For this review, take the finished solid that the model builds, in its own axes (mm). A direction names the side the tool comes from. Round coordinates to 2 decimals unless told otherwise and drop trailing zeros. Loops run counter-clockwise (first coordinate to the right, second up) from the corner with the lowest first, then second, coordinate; pieces in that order, holes last.
1. To check wall thickness, follow line 1 along Y through (x, z) = (-15.5, 0.2); line 2 along Y through (x, z) = (-35, 1.4); line 3 along X through (y, z) = (-39.5, 1.95). State the ranges of each line that lie inside material, in increasing order.
2. Clearance check with a flat-ended pin moving along its axis: pin 1 Ø1 at (x, z) = (34, 0.5) entering from +Y. State where the tip first meets the part, or that it passes through.
3. Tool access review of faces 1 (the flat face through (-69, 24.134, 2)), 2 (the cylindrical face through (-3.96, 39.67, 1.57)): name each direction out of +Z, -Z, +X, -X, +Y, -Y from which nothing blocks a thin tool from reaching the whole face with its end or side.
4. Consider section C-C on x = 26. State the section outline as (y, z) points (3 decimals), then the cut area to 3 significant figures.
5. Consider section D-D on y = 28. State the section outline as (x, z) points (3 decimals), then the cut area to 3 significant figures.
6. Draft analysis for pull direction Y (two halves, no side actions). For faces 3 (the cylindrical face through (49.284, -2.851, 1.565)), 4 (the flat face through (2, -1, 0)), 5 (the cylindrical face through (-53.986, 22.745, 1.565)), state which applies: released by +Y, released by -Y, zero draft, split by the parting line, or undercut.
7. Consider section B-B on z = 2.4. State how many separate pieces and enclosed holes the cut face has, then the cut area to 3 significant figures.
8. Consider section A-A on y = -7. State the section outline as (x, z) points (3 decimals).
from build123d import *

# Parameters (mm, degrees)
SKETCH1_R           = 64.5
SKETCH1_R_2         = 1.65
SKETCH1_R_3         = 13
SKETCH1_R_4         = 1.4
BOSS_EXTRUDE2_DEPTH = 3.175
CUT_EXTRUDE1_DEPTH  = 3.175


with BuildPart() as part:
    # Sketch1 → Boss-Extrude2 (new body)
    with BuildSketch(Plane(origin=(0, 0, 0), x_dir=(-1, 0, 0), z_dir=(0, 0, 1))):
        with Locations((15.168596538, 0.366425758)):
            Circle(SKETCH1_R)
        with Locations((15.168596538, -60.283574242)):
            Circle(SKETCH1_R_2, mode=Mode.SUBTRACT)
        with Locations((15.168596538, 61.016425758)):
            Circle(SKETCH1_R_2, mode=Mode.SUBTRACT)
        with Locations((26.018596538, -38.058574242)):
            Circle(SKETCH1_R_2, mode=Mode.SUBTRACT)
        with Locations((4.318596538, -38.058574242)):
            Circle(SKETCH1_R_2, mode=Mode.SUBTRACT)
        with Locations((26.018596538, 38.791425758)):
            Circle(SKETCH1_R_2, mode=Mode.SUBTRACT)
        with Locations((4.318596538, 38.791425758)):
            Circle(SKETCH1_R_2, mode=Mode.SUBTRACT)
        with Locations((15.168596538, 0.366425758)):
            Circle(SKETCH1_R_3, mode=Mode.SUBTRACT)
        with Locations((54.168596538, -24.133574242)):
            Circle(SKETCH1_R_4, mode=Mode.SUBTRACT)
        with Locations((54.168596538, 24.866425758)):
            Circle(SKETCH1_R_4, mode=Mode.SUBTRACT)
        with Locations((-3.831403462, -24.133574242)):
            Circle(SKETCH1_R_4, mode=Mode.SUBTRACT)
        with Locations((-3.831403462, 24.866425758)):
            Circle(SKETCH1_R_4, mode=Mode.SUBTRACT)
        with Locations((-5.831403462, 56.366425758)):
            Circle(SKETCH1_R_2, mode=Mode.SUBTRACT)
        with Locations((-22.394874657, 46.366425758)):
            Circle(SKETCH1_R_2, mode=Mode.SUBTRACT)
        with Locations((36.168596538, 56.366425758)):
            Circle(SKETCH1_R_2, mode=Mode.SUBTRACT)
        with Locations((52.732067734, 46.366425758)):
            Circle(SKETCH1_R_2, mode=Mode.SUBTRACT)
        with Locations((52.732067734, -45.633574242)):
            Circle(SKETCH1_R_2, mode=Mode.SUBTRACT)
        with Locations((36.168596538, -55.633574242)):
            Circle(SKETCH1_R_2, mode=Mode.SUBTRACT)
        with Locations((-5.831403462, -55.633574242)):
            Circle(SKETCH1_R_2, mode=Mode.SUBTRACT)
        with Locations((-22.394874657, -45.633574242)):
            Circle(SKETCH1_R_2, mode=Mode.SUBTRACT)
    extrude(amount=BOSS_EXTRUDE2_DEPTH)

    # Sketch2 → Cut-Extrude1 (cut)
    with BuildSketch(Plane.XY.offset(3.175)):
        with BuildLine():
            Line((-74.834332099, 24.133574242), (-62.834332099, 24.133574242))
            Line((-62.834332099, 24.133574242), (-62.834332099, -24.866425758))
            Line((-62.834332099, -24.866425758), (-74.834332099, -24.866425758))
            ThreePointArc((-74.834332099, -24.866425758), (-79.668596538, -0.366425758), (-74.834332099, 24.133574242))
        make_face()
    extrude(amount=-CUT_EXTRUDE1_DEPTH, mode=Mode.SUBTRACT)


solid = part.part
Resolved:
1. line 1: y = -64.87 to -62.63, -59.4 to -13.36, 12.63 to 58.67, 61.9 to 64.13
1. line 2: y = -61.74 to -57.53, -55.2 to 54.47, 56.8 to 61.01
1. line 3: x = -66.44 to -27.51, -24.53 to -5.81, -2.83 to 36.1
2. pin 1: stops at y = 41.96
3. face 1: +Z, -Z, -X
3. face 2: +Z, -Z
4. outline: (-50.019, 0) - (49.286, 0) - (49.286, 3.175) - (-50.019, 3.175) - close
4. area: 315 mm2
5. outline: (-73.096, 0) - (42.759, 0) - (42.759, 3.175) - (-73.096, 3.175) - close
5. area: 368 mm2
6. face 3: split by the parting line
6. face 4: zero draft
6. face 5: undercut
7. separate pieces: 1
7. enclosed holes: 19
7. area: 11,600 mm2
8. outline: (-62.834, 0) - (-26.349, 0) - (-26.349, 3.175) - (-62.834, 3.175) - close; (-3.988, 0) - (48.989, 0) - (48.989, 3.175) - (-3.988, 3.175) - close
